Work out the finished part from the listing and answer in its coordinate system (mm). A direction names the side the tool comes from. Coordinates: 2 decimals unless noted, no trailing zeros. Write each loop counter-clockwise with the first axis right and the second up, starting at its lowest first coordinate (ties: lowest second). Pieces come first, ordered by that corner, then holes. Notation, with made-up numbers: (13.25, 17) - (41.25, 17) arc R21 ccw to (41.25, 52) - close; hole circle Ø1 at (69, 80.5). An arc over 180 degrees is marked (long way). Answer as a JSON object with one key per item and string values. Group by question number.
from build123d import *

# Parameters (mm, degrees)
SKETCH1_W           = 90
SKETCH1_H           = 60
BOSS_EXTRUDE1_DEPTH = 10
SKETCH2_W           = 90
SKETCH2_H           = 10
BOSS_EXTRUDE2_DEPTH = 60
SKETCH3_W           = 25
SKETCH3_H           = 15
CUT_EXTRUDE1_DEPTH  = 10
SKETCH5_W           = 15
SKETCH5_H           = 15
CUT_EXTRUDE2_DEPTH  = 10
RIB1_REACH          = 119.898
SKETCH6_WALL_W      = 301.827764826
SKETCH6_WALL_H      = 10


with BuildPart() as part:
    # Sketch1 → Boss-Extrude1 (new body)
    with BuildSketch(Plane(origin=(0, 0, 0), x_dir=(1, 0, 0), z_dir=(0, 1, 0))):
        Rectangle(SKETCH1_W, SKETCH1_H)
    extrude(amount=BOSS_EXTRUDE1_DEPTH)

    # Sketch2 → Boss-Extrude2 (add)
    with BuildSketch(Plane(origin=(0, 10, 0), x_dir=(1, 0, 0), z_dir=(0, 1, 0))):
        with Locations((0, 25)):
            Rectangle(SKETCH2_W, SKETCH2_H)
    extrude(amount=BOSS_EXTRUDE2_DEPTH)

    # Sketch3 → Cut-Extrude1 (cut)
    with BuildSketch(Plane.XY.offset(-20)):
        with Locations((0, 40)):
            Rectangle(SKETCH3_W, SKETCH3_H)
    extrude(amount=-CUT_EXTRUDE1_DEPTH, mode=Mode.SUBTRACT)

    # Sketch5 → Cut-Extrude2 (cut)
    with BuildSketch(Plane(origin=(0, 10, 0), x_dir=(1, 0, 0), z_dir=(0, 1, 0))):
        Rectangle(SKETCH5_W, SKETCH5_H)
    extrude(amount=-CUT_EXTRUDE2_DEPTH, mode=Mode.SUBTRACT)

    # Sketch6 wall → Rib1 (add, up to next)
    with BuildSketch(Plane(origin=(-45, 35, 0), x_dir=(0, 0.780868809443, -0.624695047554), z_dir=(0, -0.624695047554, -0.780868809443)), mode=Mode.PRIVATE) as rib1_sk1:
        with Locations((0, 5)):
            Rectangle(SKETCH6_WALL_W, SKETCH6_WALL_H)
    rib1_tool1 = extrude(rib1_sk1.sketch, amount=RIB1_REACH, mode=Mode.PRIVATE) - part.part
    rib1 = rib1_tool1.solids().sort_by_distance((-45, 35, 0))[0]
    add(rib1)

    # Mirror1: Rib1 across plane
    add(rib1.mirror(Plane(origin=(0, 0, 0), x_dir=(0, 0, 1), z_dir=(1, 0, 0))))


solid = part.part
Q1. Flat-ended cylindrical pins translate along their axes: pin 1 Ø10 at (y, z) = (34, 3) entering from -X; pin 2 Ø5 at (x, y) = (17.5, 36.5) entering from +Z; pin 3 Ø3 at (x, z) = (-15.5, -6) entering from +Y. Find the tip coordinate at first contact, or state that the pin passes through.
Q2. Section D-D on z = 16 is taken. Determine the outline of the cut face in (x, y).
Q3. For a pull along Y with two mould halves and no side action, classify faces 5 (the face through (12.5, 40, -25)), 6 (the face through (-1, 10, 10)), 7 (the face through (-12.5, 40, -25)), 8 (the face through (-1, 53, -20)) as +Y half, -Y half, draft (parallel to the pull), parting line (faces both ways), or undercut.
Q4. Section B-B on y = 57 is taken. Determine the outline of the cut face in (x, z), plus the area to 3 significant figures.
Q5. Section A-A on x = 5 is taken. Determine the outline of the cut face in (y, z).
Q6. Section C-C on z = 3.5 is taken. Determine the outline of the cut face in (x, y) (3 decimals).
Q7. Consider L1, parallel to X at y = 22, z = -17.5; L2, parallel to Z at x = -15, y = 47; L3, parallel to Y at x = -30, z = 27. Determine where each line is inside the solid, lowest interval first. Write a range as from..to.
Q8. A tool of negligible diameter and unlimited length cuts with its end or side. For faces 1 (the face through (7.5, 5, 0)), 2 (the face through (0, 47.5, -25)), 3 (the face through (45, 27, -9)), 4 (the face through (35, 27, -9)), from which of +Z, -Z, +X, -X, +Y, -Y can it reach the whole face along a straight path? Write none if from no direction.
Numbers:
{
 "1": {"pin 1": "stops at x = -45", "pin 2": "stops at z = -20", "pin 3": "stops at y = 10"},
 "2": {"outline": "(-45, 0) - (45, 0) - (45, 15) - (35, 15) - (35, 10) - (-35, 10) - (-35, 15) - (-45, 15) - close"},
 "3": {"face 5": "undercut", "face 6": "+Y half", "face 7": "undercut", "face 8": "draft"},
 "4": {"outline": "(-45, -30) - (45, -30) - (45, -17.6) - (35, -17.6) - (35, -20) - (-35, -20) - (-35, -17.6) - (-45, -17.6) - close", "area": "948 mm²"},
 "5": {"outline": "(0, -30) - (32.5, -30) - (32.5, -20) - (10, -20) - (10, -7.5) - (0, -7.5) - close; (0, 7.5) - (10, 7.5) - (10, 30) - (0, 30) - close; (47.5, -30) - (70, -30) - (70, -20) - (47.5, -20) - close"},
 "6": {"outline": "(-45, 0) - (-7.5, 0) - (-7.5, 10) - (-35, 10) - (-35, 30.625) - (-45, 30.625) - close; (7.5, 0) - (45, 0) - (45, 30.625) - (35, 30.625) - (35, 10) - (7.5, 10) - close"},
 "7": {"L1": "x = -45..-35, 35..45", "L2": "z = -30..-20", "L3": "y = 0..10"},
 "8": {"face 1": "+Y, -Y", "face 2": "+Z, -Z", "face 3": "+Z, -Z, +X, +Y, -Y", "face 4": "+Z, +Y"}
}
